Build history of the part. All positions in model axes, mm. Face numbers are marked on the shaded views. A direction names the side the tool comes from. Coordinates: 2 decimals unless noted, no trailing zeros. Loops run counter-clockwise (first coordinate to the right, second up) from the corner with the lowest first, then second, coordinate; pieces in that order, holes last. Notation, with made-up numbers: (-4.75, 13) - (23.25, 13) arc R13 ccw to (23.25, 19) - close; hole circle Ø8 at (-2, -30.5). An arc over 180 degrees is marked (long way). One line per item, written item: value.
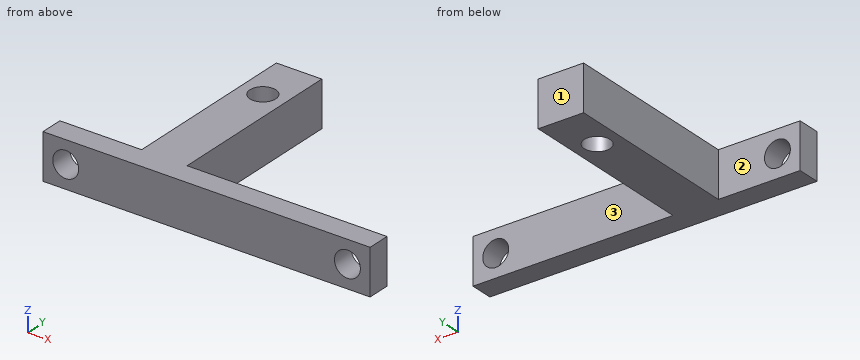
```python
from build123d import *

# Parameters (mm, degrees)
SKETCH1_W           = 54.864
SKETCH1_H           = 7.62
BOSS_EXTRUDE1_DEPTH = 3.81
SKETCH2_R           = 2.1717
CUT_EXTRUDE2_DEPTH  = 3.81
SKETCH5_W           = 7.62
SKETCH5_H           = 7.62
BOSS_EXTRUDE2_DEPTH = 30.48
SKETCH6_R           = 2.1717
CUT_EXTRUDE3_DEPTH  = 7.62


with BuildPart() as part:
    # Sketch1 → Boss-Extrude1 (new body)
    with BuildSketch(Plane(origin=(0, 0, 0), x_dir=(1, 0, 0), z_dir=(0, 1, 0))):
        with Locations((2.806390244, -28.85997561)):
            Rectangle(SKETCH1_W, SKETCH1_H)
    extrude(amount=BOSS_EXTRUDE1_DEPTH)

    # Sketch2 → Cut-Extrude2 (cut)
    with BuildSketch(Plane(origin=(0, 3.81, 0), x_dir=(1, 0, 0), z_dir=(0, 1, 0))):
        with Locations(Location((-20.815609756, -28.85997561, 0), (0, 0, 270))):
            Circle(SKETCH2_R)
        with Locations(Location((26.428390244, -28.85997561, 0), (0, 0, 270))):
            Circle(SKETCH2_R)
    extrude(amount=-CUT_EXTRUDE2_DEPTH, mode=Mode.SUBTRACT)

    # Sketch5 → Boss-Extrude2 (add)
    with BuildSketch(Plane(origin=(0, 3.81, 0), x_dir=(1, 0, 0), z_dir=(0, 1, 0))):
        with Locations((-7.099609756, -28.85997561)):
            Rectangle(SKETCH5_W, SKETCH5_H)
    extrude(amount=BOSS_EXTRUDE2_DEPTH)

    # Sketch6 → Cut-Extrude3 (cut)
    with BuildSketch(Plane.XY.offset(32.66997561)):
        with Locations((-7.099609756, 26.0985)):
            Circle(SKETCH6_R)
    extrude(amount=-CUT_EXTRUDE3_DEPTH, mode=Mode.SUBTRACT)


solid = part.part
```
Item 1: Tool access for the marked faces 1, 2 and 3: list every direction of +Z, -Z, +X, -X, +Y, -Y with a clear straight run to the whole face (end or side of a thin tool).
Check result:
face 1: +Z, -Z, +X, -X, +Y
face 2: +Z, -Z, -X, +Y
face 3: +Z, -Z, +X, +Y
Item 2: Probe probe 1 along X at (y, z) = (2, 29); probe 2 along X at (y, z) = (16, 29.5); probe 3 along Y at (x, z) = (11, 32). List the from-to ranges inside material, lowest first. Write a range as from..to.
Check result:
probe 1: x = -24.63..-22.98, -18.65..24.26, 28.6..30.24
probe 2: x = -10.91..-3.29
probe 3: y = 0..3.81
Item 3: Cut at D-D, the plane y = 11. Write the cut outline in (x, z), then the cut area to 3 significant figures.
Check result:
outline: (-10.91, 25.05) - (-3.29, 25.05) - (-3.29, 32.67) - (-10.91, 32.67) - close
area: 58.1 mm^2
Item 4: Cut at A-A, the plane z = 28.75. Write the cut outline in (x, y), then the cut area to 3 significant figures.
Check result:
outline: (-24.63, 0) - (-22.98, 0) - (-22.98, 3.81) - (-24.63, 3.81) - close; (-18.65, 0) - (24.26, 0) - (24.26, 3.81) - (-3.29, 3.81) - (-3.29, 34.29) - (-10.91, 34.29) - (-10.91, 3.81) - (-18.65, 3.81) - close; (28.6, 0) - (30.24, 0) - (30.24, 3.81) - (28.6, 3.81) - close; hole circle Ø4.34 at (-7.1, 26.1)
area: 393 mm^2
Item 5: Cut at B-B, the plane x = -20. Write the cut outline in (y, z).
Check result:
outline: (0, 25.05) - (3.81, 25.05) - (3.81, 26.85) - (0, 26.85) - close; (0, 30.87) - (3.81, 30.87) - (3.81, 32.67) - (0, 32.67) - close
Item 6: Cut at C-C, the plane z = 31.75. Write the cut outline in (x, y), then the cut area to 3 significant figures.
Check result:
outline: (-24.63, 0) - (30.24, 0) - (30.24, 3.81) - (-3.29, 3.81) - (-3.29, 34.29) - (-10.91, 34.29) - (-10.91, 3.81) - (-24.63, 3.81) - close; hole circle Ø4.34 at (-7.1, 26.1)
area: 426 mm^2
Item 7: Drop flat-ended pins along their axis: P1, Ø1.5, axis at y = 13.5, z = 29.5, coming from the +X side; P2, Ø1.5, axis at y = 14, z = 31.5, coming from the -X side. Give the stop position or say it passes through.
Check result:
P1: stops at x = -3.29
P2: stops at x = -10.91
